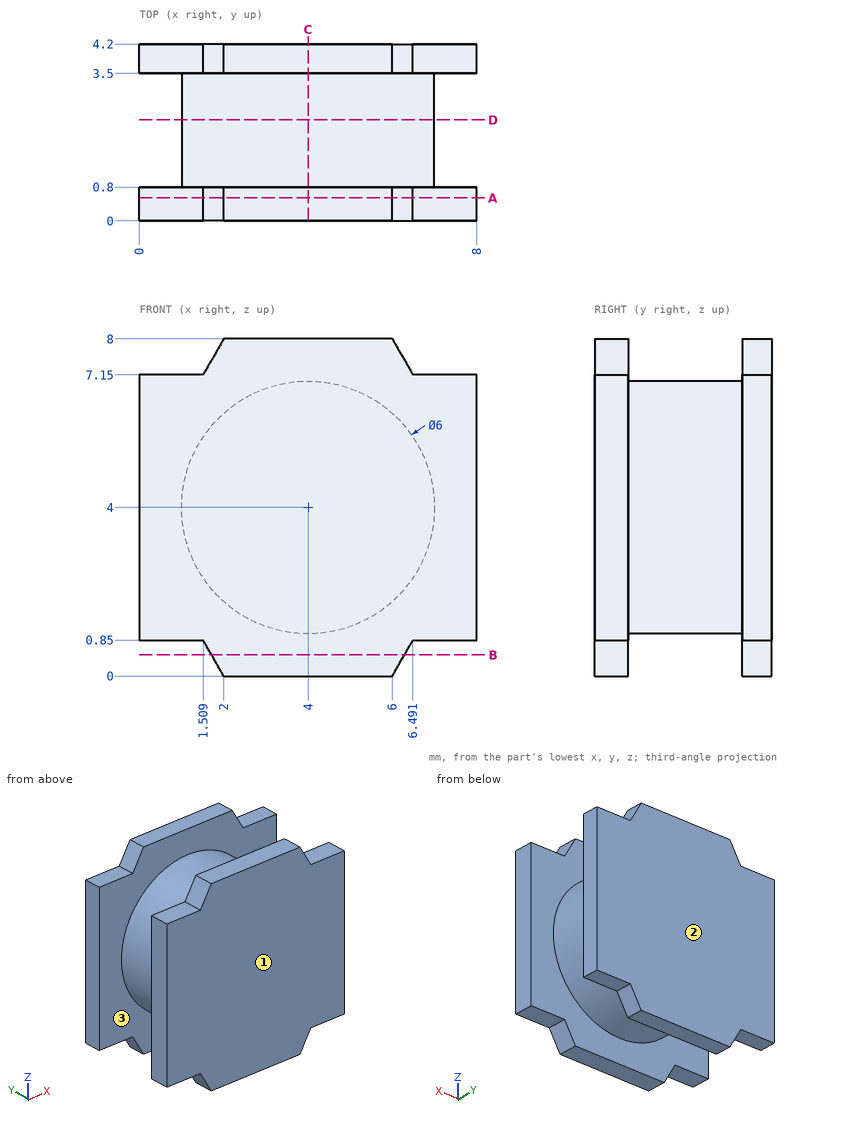
Input: dimensioned drawing with shaded views. Units: mm. Origin: part minimum x, y, z. Coordinates: 2 decimals unless noted, no trailing zeros. Loops run counter-clockwise (first coordinate to the right, second up) from the corner with the lowest first, then second, coordinate; pieces in that order, holes last. Notation, with made-up numbers: (61, 13.5) -> (71, 13.5) arc R20 cw to (71, 31.5) -> close; hole circle Ø3 at (60.25, 77.25). An arc over 180 degrees is marked (long way). One line per item, written item: value. Start each with the question number.
Q1. Section query D-D, the plane y = 2.4. Return the cut outline in (x, z), and give its area (3 significant figures).
Q2. Section query A-A, the plane y = 0.55. Return the cut outline in (x, z).
Q3. Contact query for flat-ended pins moving along their axis: P1, Ø0.8, axis at x = 0.5, y = 4, coming from the -Z side; P2, Ø0.9, axis at x = 0.5, y = 0.5, coming from the +Z side. Output: stop coordinate, or through.
Q4. Section query B-B, the plane z = 0.5. Return the cut outline in (x, y).
Q5. Line query: line 1 along Y through (x, z) = (4.5, 7.5); line 2 along Z through (x, y) = (1, 3.65); line 3 along Z through (x, y) = (2, 1.6) (1 decimal). Output: solid intervals per line, ascending.
Q6. Mould query, pull axis Y, two halves, no side actions, for the marked faces 1, 2 and 3. Classes: pulls with the +Y half, pulls with the -Y half, needs draft (parallel to the pull), parting line crosses it, or undercut.
Q7. Section query C-C, the plane x = 4. Return the cut outline in (y, z), and give its area (3 significant figures).
Results:
1. outline: circle Ø6 at (4, 4)
1. area: 28.3 mm^2
2. outline: (0, 0.85) -> (1.51, 0.85) -> (2, 0) -> (6, 0) -> (6.49, 0.85) -> (8, 0.85) -> (8, 7.15) -> (6.49, 7.15) -> (6, 8) -> (2, 8) -> (1.51, 7.15) -> (0, 7.15) -> close
3. P1: z = 0.85
3. P2: z = 7.15
4. outline: (1.71, 0) -> (6.29, 0) -> (6.29, 0.8) -> (1.71, 0.8) -> close; (1.71, 3.5) -> (6.29, 3.5) -> (6.29, 4.2) -> (1.71, 4.2) -> close
5. line 1: 0 to 0.8, 3.5 to 4.2
5. line 2: 0.85 to 7.15
5. line 3: 1.8 to 6.2
6. face 1: pulls with the -Y half
6. face 2: pulls with the +Y half
6. face 3: undercut
7. outline: (0, 0) -> (0.8, 0) -> (0.8, 1) -> (3.5, 1) -> (3.5, 0) -> (4.2, 0) -> (4.2, 8) -> (3.5, 8) -> (3.5, 7) -> (0.8, 7) -> (0.8, 8) -> (0, 8) -> close
7. area: 28.2 mm^2
